For this review, take the finished solid that the model builds, in its own axes (mm). Face numbers are marked on the shaded views. A direction names the side the tool comes from. Give positions to 0.01 mm unless a question says otherwise; leave off trailing zeros. Loops run counter-clockwise (first coordinate to the right, second up) from the corner with the lowest first, then second, coordinate; pieces in that order, holes last. Notation, with made-up numbers: (6, 38.5) - (45, 38.5) arc R27 cw to (45, 66.5) - close; hole circle Ø6 at (10.5, 75.25). An arc over 180 degrees is marked (long way). Put each result on its own line as item: value.
from build123d import *

# Parameters (mm, degrees)
SKETCH1_W           = 6.35
SKETCH1_H           = 107.95
BOSS_EXTRUDE1_DEPTH = 31.75
BOSS_EXTRUDE2_DEPTH = 19.304
SKETCH3_W           = 63.5
SKETCH3_H           = 47.625
BOSS_EXTRUDE3_DEPTH = 3.175
SKETCH5_R           = 2.54
CUT_EXTRUDE2_DEPTH  = 23.479
FILLET1_R           = 2.54
CUT_EXTRUDE4_START  = -6.35
SKETCH7_W           = 50.8
SKETCH7_H           = 19.304
CUT_EXTRUDE4_DEPTH  = 6.35
SKETCH9_R           = 2.25
CUT_EXTRUDE5_DEPTH  = 23.479
SKETCH15_R          = 2.55
SKETCH15_R_2        = 5.175
CUT_EXTRUDE8_DEPTH  = 23.479
LPATTERN1_COUNT     = 3
LPATTERN1_PITCH     = 12.7


with BuildPart() as part:
    # Sketch1 → Boss-Extrude1 (new body, symmetric)
    with BuildSketch(Plane(origin=(0, 0, 0), x_dir=(0, 0, -1), z_dir=(1, 0, 0))):
        with Locations((3.175, 0)):
            Rectangle(SKETCH1_W, SKETCH1_H)
    extrude(amount=BOSS_EXTRUDE1_DEPTH, both=True)

    # Sketch2 → Boss-Extrude2 (add)
    with BuildSketch(Plane.XY):
        Polygon((-31.75, 53.975), (-31.75, 101.6), (-25.4, 101.6), (25.4, 101.6), (31.75, 101.6), (31.75, 53.975), (25.4, 53.975), (25.4, 95.25), (-25.4, 95.25), (-25.4, 53.975), align=None)
    extrude(amount=-BOSS_EXTRUDE2_DEPTH)

    # Sketch3 → Boss-Extrude3 (add)
    with BuildSketch(Plane(origin=(0, 0, -19.304), x_dir=(-1, 0, 0), z_dir=(0, 0, -1))):
        with Locations((0, 77.7875)):
            Rectangle(SKETCH3_W, SKETCH3_H)
    extrude(amount=BOSS_EXTRUDE3_DEPTH)

    # Sketch5 → Cut-Extrude2 (cut, through all)
    with BuildSketch(Plane(origin=(0, 0, -22.479), x_dir=(-1, 0, 0), z_dir=(0, 0, -1))):
        with Locations((15.5, 94.425)):
            Circle(SKETCH5_R)
        with Locations((15.5, 63.425)):
            Circle(SKETCH5_R)
        with Locations((-15.5, 63.425)):
            Circle(SKETCH5_R)
        with Locations((-15.5, 94.425)):
            Circle(SKETCH5_R)
        with BuildLine():
            Line((-11.1125, 87.905256121), (-11.1125, 101.6))
            Line((-11.1125, 101.6), (11.1125, 101.6))
            Line((11.1125, 101.6), (11.1125, 87.905256121))
            ThreePointArc((11.1125, 87.905256121), (0, 64.6375), (-11.1125, 87.905256121))
        make_face()
    extrude(amount=-CUT_EXTRUDE2_DEPTH, mode=Mode.SUBTRACT)

    # Fillet1
    fillet1_edges = [part.edges().sort_by_distance(p)[0] for p in [
        (-31.75, 101.6, -11.2395),
        (31.75, 101.6, -11.2395),
        (-11.1125, 87.905256121, -20.8915),
        (11.1125, 87.905256121, -20.8915),
        (11.1125, 101.6, -11.2395),
        (-11.1125, 101.6, -11.2395),
    ]]
    fillet(fillet1_edges, radius=FILLET1_R)

    # Sketch7 → Cut-Extrude4 (cut)
    with BuildSketch(Plane(origin=(0, 101.6, 0), x_dir=(1, 0, 0), z_dir=(0, 1, 0)).offset(CUT_EXTRUDE4_START)):
        with Locations((0, 9.652)):
            Rectangle(SKETCH7_W, SKETCH7_H)
    extrude(amount=CUT_EXTRUDE4_DEPTH, mode=Mode.SUBTRACT)

    # Sketch9 → Cut-Extrude5 (cut, through all)
    with BuildSketch(Plane.XY):
        with Locations((25.4, -47.625)):
            Circle(SKETCH9_R)
        with Locations((-25.4, -47.625)):
            Circle(SKETCH9_R)
    cut_extrude5 = extrude(amount=-CUT_EXTRUDE5_DEPTH, mode=Mode.SUBTRACT)

    # Sketch15 → Cut-Extrude8 (cut, through all)
    with BuildSketch(Plane.XY):
        with Locations((10, 72.981043446)):
            Circle(SKETCH15_R)
        with Locations((-10, 33.281043446)):
            Circle(SKETCH15_R)
        with Locations((-10, 72.981043446)):
            Circle(SKETCH15_R)
        with Locations((10, 33.281043446)):
            Circle(SKETCH15_R)
        with Locations((-20, 72.981043446)):
            Circle(SKETCH15_R_2)
        with Locations((20, 72.981043446)):
            Circle(SKETCH15_R_2)
        with Locations((20, 32.981043446)):
            Circle(SKETCH15_R_2)
        with Locations((-20, 32.981043446)):
            Circle(SKETCH15_R_2)
    extrude(amount=-CUT_EXTRUDE8_DEPTH, mode=Mode.SUBTRACT)

    # LPattern1: Cut-Extrude5 ×3
    with Locations(*[(0, i * LPATTERN1_PITCH, 0) for i in range(1, LPATTERN1_COUNT)]):
        add(cut_extrude5, mode=Mode.SUBTRACT)


solid = part.part
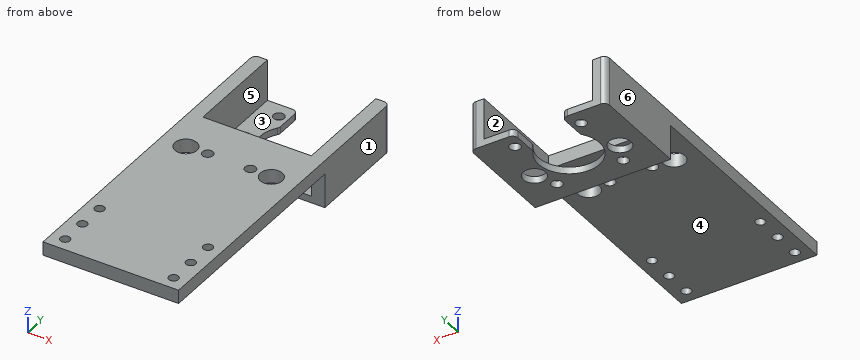
1) Insertion check: pin 1 Ø19 at (x, y) = (6, -11) entering from -Z; pin 2 Ø3 at (x, z) = (10.5, -19) entering from +Y; pin 3 Ø4 at (x, z) = (24.5, -18.5) entering from -Y (3 decimals); pin 4 Ø6 at (x, z) = (22, -10.5) entering from +Y. Each pin has a flat end and moves straight along its axis. Give the tip position at first contact, or say it passes through.
Geometry check:
pin 1: stops at z = -6.35
pin 2: stops at y = 100.96
pin 3: stops at y = 53.975
pin 4: passes through
2) Take a section at D-D on z = -20.75. State how many separate pieces and enclosed holes the cut face has, and give its area (3 significant figures).
Geometry check:
separate pieces: 1
enclosed holes: 6
area: 1,910 mm²
3) Take a section at C-C on y = 74.5. State the section outline as (x, z) points (3 decimals), and give its area (3 significant figures).
Geometry check:
outline: (-31.75, -22.479) - (-24.947, -22.479) - (-24.947, -19.304) - (-25.4, -19.304) - (-25.4, 0) - (-31.75, 0) - close; (-15.053, -22.479) - (-13.585, -22.479) - (-13.585, -19.304) - (-15.053, -19.304) - close; (13.585, -22.479) - (15.053, -22.479) - (15.053, -19.304) - (13.585, -19.304) - close; (24.947, -22.479) - (31.75, -22.479) - (31.75, 0) - (25.4, 0) - (25.4, -19.304) - (24.947, -19.304) - close
area: 298 mm²
4) Wall thickness on line 1 (Y direction, x = -10, z = -3) (3 decimals); line 2 (X direction, y = 37.5, z = -1.5); line 3 (X direction, y = 82.5, z = -19): over which ranges is each line inside the solid? List them lowest first.
Geometry check:
line 1: y = -53.975 to 30.731, 35.831 to 53.975
line 2: x = -31.75 to -22.52, -17.48 to 17.48, 22.52 to 31.75
line 3: x = -31.75 to -25.4, 25.4 to 31.75
5) Draft analysis for pull direction X (two halves, no side actions). For the marked faces 4, 5 and 6, state which applies: pulls with the +X half, pulls with the -X half, needs draft (parallel to the pull), parting line crosses it, or undercut.
Geometry check:
face 4: needs draft
face 5: undercut
face 6: pulls with the -X half
6) Take a section at A-A on z = -9.25. State the section outline as (x, y) points (3 decimals), and give its area (3 significant figures).
Geometry check:
outline: (-31.75, 53.975) - (-25.4, 53.975) - (-25.4, 101.6) - (-29.21, 101.6) arc R2.54 ccw to (-31.75, 99.06) - close; (25.4, 53.975) - (31.75, 53.975) - (31.75, 99.06) arc R2.54 ccw to (29.21, 101.6) - (25.4, 101.6) - close
area: 602 mm²
7) For the marked faces 1, 2 and 3, list the 3-axis set-ups (+Z, -Z, +X, -X, +Y, -Y) from which the entire face can be reached by the end or side of a thin tool; tool diameter is ignored.
Geometry check:
face 1: +Z, -Z, +X, +Y, -Y
face 2: +Z, +Y
face 3: +Z, +Y, -Y
